Check sheet for the drawn part. Datum: minimum x, y, z corner. Units: mm. Give positions to 0.01 mm unless a question says otherwise; leave off trailing zeros. Order: outer loops, then holes, each group sorted by start corner. A loop starts at its lowest first (then second) coordinate and runs counter-clockwise, first axis right, second up.
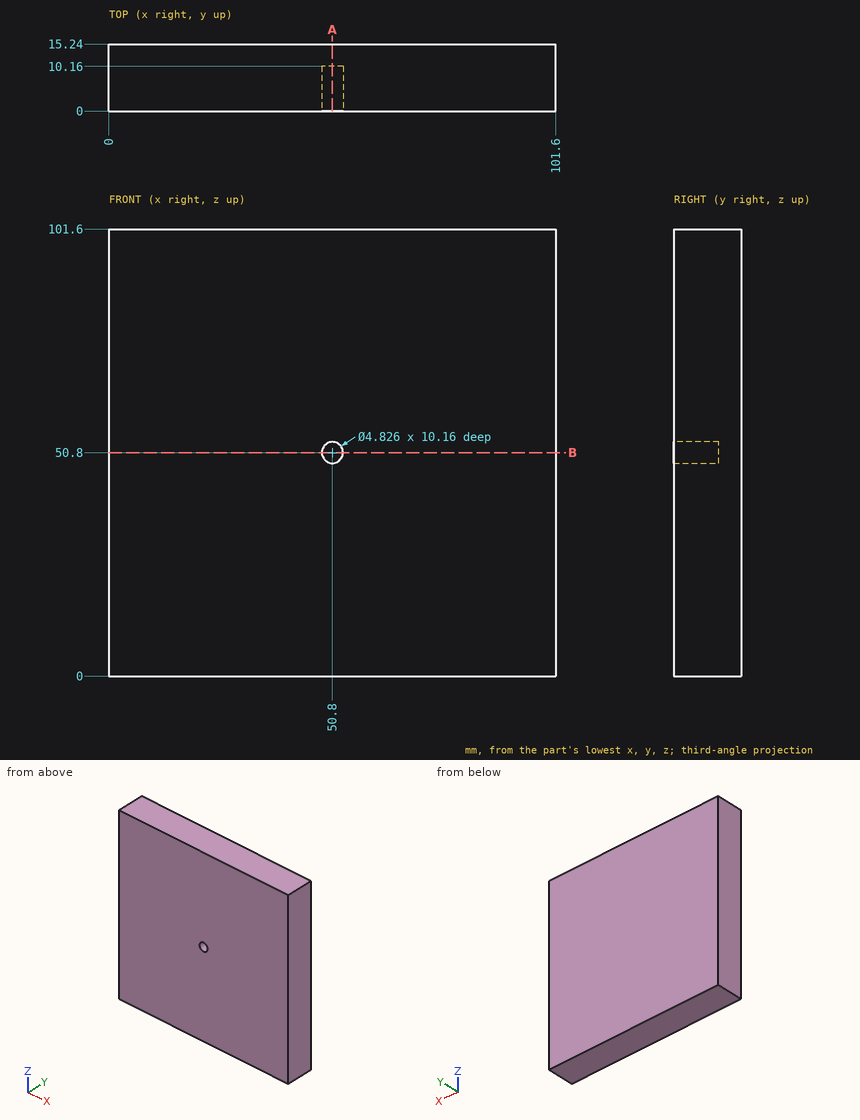
Item 1: Sectioned sample at B-B (z = 50.8). Enter the section's corners in (x, y).
Reported:
outline: (0, 0) - (48.39, 0) - (48.39, 10.16) - (53.21, 10.16) - (53.21, 0) - (101.6, 0) - (101.6, 15.24) - (0, 15.24) - close
Item 2: Gauge pin test, flat end, axial feed: pin 1 (1.5 mm diameter, centred on x = 29.5, y = 7, fed in from -Z). Record the tip position at first contact, or that the pin passes through.
Reported:
pin 1: stops at z = 0
Item 3: Scan lines: L1, parallel to X at y = 6.75, z = 50.8; L2, parallel to Z at x = 51.5, y = 1. Record each from-to range of solid material in increasing order.
Reported:
L1: x = 0 to 48.39, 53.21 to 101.6
L2: z = 0 to 48.49, 53.11 to 101.6
Item 4: Sectioned sample at A-A (x = 50.8). Enter the section's corners in (y, z).
Reported:
outline: (0, 0) - (15.24, 0) - (15.24, 101.6) - (0, 101.6) - (0, 53.21) - (10.16, 53.21) - (10.16, 48.39) - (0, 48.39) - close
